Can you work these out from the drawing? Everything is in mm from the part's minimum corner. Coordinates: 2 decimals unless noted, no trailing zeros. Answer in a Markdown table with one row per item.
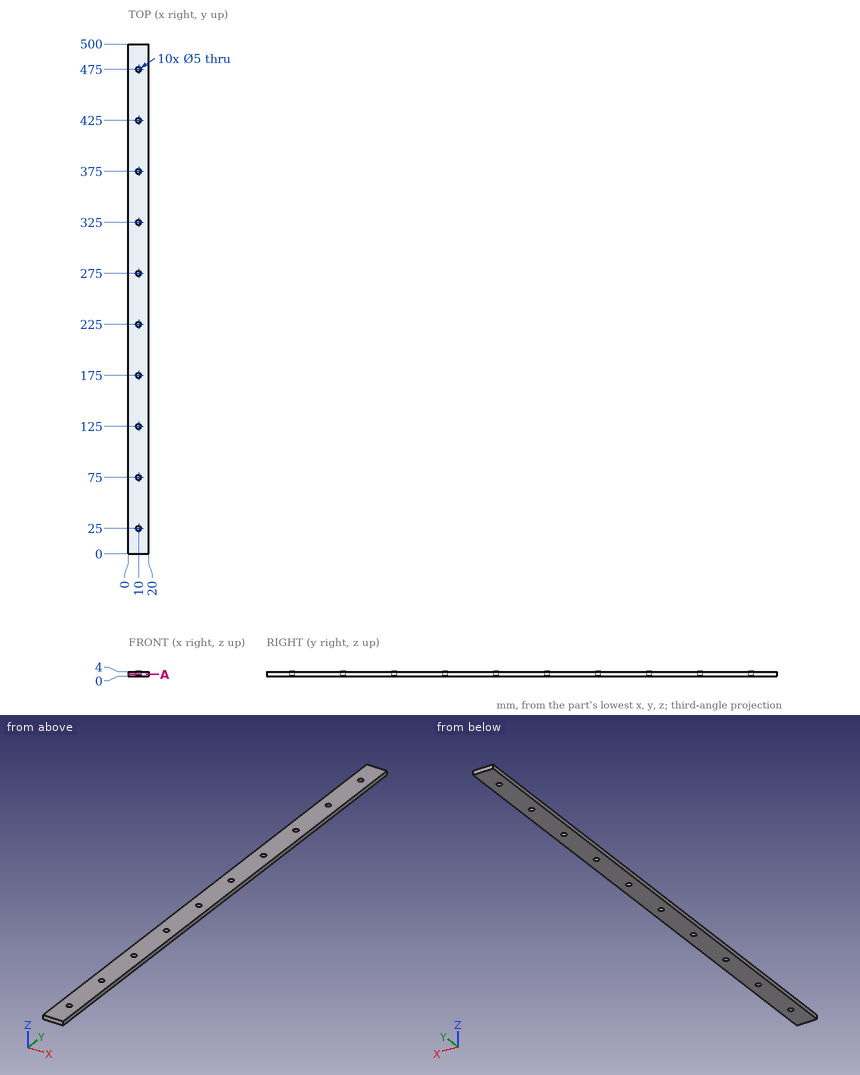
(1) Will this pin go through, and if not, where does the flat tip stop? pin 1 Ø4 at (x, y) = (10, 225) entering from +Z.
Response values:
| item | result |
|---|---|
| pin 1 | through |
(2) I need wall thicknesses on line 1 (X direction, y = 375, z = 2.25). Which ranges of the line are inside material? Lowest first, please. Write a range as [from, to].
Response values:
| item | result |
|---|---|
| line 1 | [0, 7.5], [12.5, 20] |
(3) Suppose I cut it at A-A (z = 1.6). Count the separate pieces of the cut face and the enclosed holes in it, and give its area (3 significant figures).
Response values:
| item | result |
|---|---|
| separate pieces | 1 |
| enclosed holes | 10 |
| area | 9,800 mm2 |
